Autodesk Inventor part; units mm, degrees
ref_plane "YZ Plane" through (0, 0, 0) normal (1, 0, 0) x (0, 1, 0)
ref_plane "XZ Plane" through (0, 0, 0) normal (0, 1, 0) x (-1, 0, 0)
ref_plane "XY Plane" through (0, 0, 0) normal (0, 0, 1) x (1, 0, 0)
sketch "Sketch4" plane through (0, 0, 0) normal (0, 0, 1) x (1, 0, 0)
  line L0 (0, 0) -> (-40, 0)
  line L1 (-40, 0) -> (-40, 20)
  line L2 (-40, 20) -> (0, 20)
  line L3 (0, 20) -> (0, 0)
  dimension "d37" = 40
  dimension "d38" = 20
extrude "Extrusion2" add sketch "Sketch4" along normal blind 10
hole "Hole2" at (-20, 10, 10) direction (0, 0, -1) diameter 6.5 depth 10 tip angle 118 counterbore diameter 10.5 counterbore depth 6.5
hole "Hole3" at (-35, 10, 10) direction (0, 0, -1) diameter 4.5 depth 10 tip angle 118 counterbore diameter 7.5 counterbore depth 4
hole "Hole4" at (-5, 10, 10) direction (0, 0, -1) diameter 4.5 depth 10 tip angle 118 counterbore diameter 7.5 counterbore depth 4
properties part number "GARFO" material "Aluminium AW-7020"
Verification items for the finished model (mm, model axes). A direction names the side the tool comes from. Coordinates: 2 decimals unless noted, no trailing zeros. Loops run counter-clockwise (first coordinate to the right, second up) from the corner with the lowest first, then second, coordinate; pieces in that order, holes last. Notation, with made-up numbers: (-2, 83.5) -> (38, 83.5) arc R20 ccw to (38, 98.5) -> close; hole circle Ø6 at (62, 88.5). An arc over 180 degrees is marked (long way). Answer in a Markdown table with one row per item.
1) Scan lines: line 1 along X through (y, z) = (10, 7); line 2 along X through (y, z) = (10, 1.85); line 3 along Y through (x, z) = (-35, 8.4). Record each from-to range of solid material in increasing order. Write a range as from..to.
The answers:
| item | result |
|---|---|
| line 1 | x = -40..-38.75, -31.25..-25.25, -14.75..-8.75, -1.25..0 |
| line 2 | x = -40..-37.25, -32.75..-23.25, -16.75..-7.25, -2.75..0 |
| line 3 | y = 0..6.25, 13.75..20 |
2) Section check C-C (x = -5). Record the cut outline in (y, z).
The answers:
| item | result |
|---|---|
| outline | (0, 0) -> (7.75, 0) -> (7.75, 6) -> (6.25, 6) -> (6.25, 10) -> (0, 10) -> close; (12.25, 0) -> (20, 0) -> (20, 10) -> (13.75, 10) -> (13.75, 6) -> (12.25, 6) -> close |
3) Section check A-A (y = 10). Record the cut outline in (x, z), and give its area (3 significant figures).
The answers:
| item | result |
|---|---|
| outline | (-40, 0) -> (-37.25, 0) -> (-37.25, 6) -> (-38.75, 6) -> (-38.75, 10) -> (-40, 10) -> close; (-32.75, 0) -> (-23.25, 0) -> (-23.25, 3.5) -> (-25.25, 3.5) -> (-25.25, 10) -> (-31.25, 10) -> (-31.25, 6) -> (-32.75, 6) -> close; (-16.75, 0) -> (-7.25, 0) -> (-7.25, 6) -> (-8.75, 6) -> (-8.75, 10) -> (-14.75, 10) -> (-14.75, 3.5) -> (-16.75, 3.5) -> close; (-2.75, 0) -> (0, 0) -> (0, 10) -> (-1.25, 10) -> (-1.25, 6) -> (-2.75, 6) -> close |
| area | 195 mm2 |
4) Section check B-B (z = 6.5). Record the cut outline in (x, y).
The answers:
| item | result |
|---|---|
| outline | (-40, 0) -> (0, 0) -> (0, 20) -> (-40, 20) -> close; hole circle Ø7.5 at (-35, 10); hole circle Ø10.5 at (-20, 10); hole circle Ø7.5 at (-5, 10) |
5) Draft check along Y on faces 3 (the face through (-32.718, 12.976, 7.972)), 4 (the face through (-20, 20, 5)), 5 (the face through (-25, 10, 0)), 6 (the face through (-20, 0, 5)). Enter one of: released by +Y, released by -Y, zero draft, split by the parting line, or undercut.
The answers:
| item | result |
|---|---|
| face 3 | undercut |
| face 4 | released by +Y |
| face 5 | zero draft |
| face 6 | released by -Y |
6) Section check D-D (x = -20). Record the cut outline in (y, z).
The answers:
| item | result |
|---|---|
| outline | (0, 0) -> (6.75, 0) -> (6.75, 3.5) -> (4.75, 3.5) -> (4.75, 10) -> (0, 10) -> close; (13.25, 0) -> (20, 0) -> (20, 10) -> (15.25, 10) -> (15.25, 3.5) -> (13.25, 3.5) -> close |
7) Depth check by flat-ended pin: P1, Ø6, axis at x = -35, y = 10, coming from the +Z side. Enter the tip coordinate at first touch or a pass-through.
The answers:
| item | result |
|---|---|
| P1 | stops at z = 6 |
8) Access from +Z, -Z, +X, -X, +Y, -Y to the whole of each face (thin tool, end or side, straight path). Record for faces 1 (the face through (-40, 10, 5)), 2 (the face through (-16.6, 10.1, 3.5)).
The answers:
| item | result |
|---|---|
| face 1 | +Z, -Z, -X, +Y, -Y |
| face 2 | +Z |
